```python
from build123d import *

# Parameters (mm, degrees)
F0_W      = 100
F0_H      = 100
F1_DEPTH  = 2
F2_R      = 0.5
F4_W      = 80
F4_H      = 80
F5_DEPTH  = 30
F6_R      = 1
F7_R      = 1
F8_W      = 50
F8_H      = 50
F9_DEPTH  = 20
F10_R     = 1
F11_W     = 40
F11_H     = 40
F12_DEPTH = 42


with BuildPart() as f1:
    # F0 (on Top) → F1 (new body)
    with BuildSketch(Plane.XY):
        Rectangle(F0_W, F0_H)
    extrude(amount=F1_DEPTH)

    # F2
    f2_edges = [f1.edges().sort_by_distance(p)[0] for p in [
        (50, 0, 2),
        (0, 50, 2),
        (-50, 0, 2),
        (0, -50, 2),
    ]]
    fillet(f2_edges, radius=F2_R)

    # F4 (on offset) → F5 (join)
    with BuildSketch(Plane.XY.offset(2)):
        Rectangle(F4_W, F4_H)
    extrude(amount=F5_DEPTH)

    # F6
    f6_edges = [f1.edges().sort_by_distance(p)[0] for p in [
        (-40, -40, 17),
        (40, -40, 17),
        (40, 40, 17),
        (-40, 40, 17),
    ]]
    fillet(f6_edges, radius=F6_R)

    # F7
    f7_edges = [f1.edges().sort_by_distance(p)[0] for p in [
        (40, 0, 32),
        (39.707107, -39.707107, 32),
        (39.707107, 39.707107, 32),
        (0, -40, 32),
        (0, 40, 32),
        (-39.707107, -39.707107, 32),
        (-39.707107, 39.707107, 32),
        (-40, 0, 32),
    ]]
    fillet(f7_edges, radius=F7_R)

    # F8 (on face) → F9 (join)
    with BuildSketch(Plane.XY.offset(32)):
        Rectangle(F8_W, F8_H)
    extrude(amount=F9_DEPTH)

    # F10
    f10_edges = [f1.edges().sort_by_distance(p)[0] for p in [
        (-25, -25, 42),
        (25, -25, 42),
        (0, -25, 32),
        (0, -25, 52),
        (-25, 25, 42),
        (-25, 0, 32),
        (-25, 0, 52),
        (25, 0, 52),
        (0, 25, 52),
        (25, 25, 42),
        (25, 0, 32),
        (0, 25, 32),
    ]]
    fillet(f10_edges, radius=F10_R)

    # F11 (on face) → F12 (cut)
    with BuildSketch(Plane(origin=(0, 0, 0), x_dir=(1, 0, 0), z_dir=(0, 0, -1))):
        Rectangle(F11_W, F11_H)
    extrude(amount=-F12_DEPTH, mode=Mode.SUBTRACT)


solid = f1.part
```
Could you check a few things on this model? Use its own coordinates, in mm. A direction names the side the tool comes from. Coordinates: 2 decimals unless noted, no trailing zeros. Order: outer loops, then holes, each group sorted by start corner. A loop starts at its lowest first (then second) coordinate and runs counter-clockwise, first axis right, second up. Notation, with made-up numbers: M 66,77.5 L 120,77.5 A6 cw 120,82.5 Z; hole C -17,-36 d3. An arc over 180 degrees is marked long. Use a Markdown table: item, result. Add a question column.
Q1. I want a section at A-A on z = 37. List the corners of the cut face in (x, y) for me.
Q2. We'd pull the mould along X, two halves only. Please class faces 6 (the flat face through (0, 20, 21)), 7 (the flat face through (0, 25, 42)), 8 (the flat face through (-25, 0, 42)): pulls with the +X half, pulls with the -X half, needs draft (parallel to the pull), parting line crosses it, or undercut.
Q3. I'm going to push flat-ended pins straight in: pin 1 (14.5 mm diameter, centred on x = 9, z = 41, fed in from -Y); pin 2 (9 mm diameter, centred on y = -8, z = 39, fed in from -X); pin 3 (23 mm diameter, centred on x = -12.5, z = 18.5, fed in from +Y). Where does each tip first touch, or does it pass through?
Q4. If I drill on L1, parallel to X at y = -9, z = 3.5; L2, parallel to X at y = 28.5, z = 12.5, over which ranges is the centre line in solid material (lowest first)?
Q5. I want a section at C-C on y = 16. List the corners of the cut face in (x, z) for me.
Q6. I want a section at B-B on x = -28. List the corners of the cut face in (y, z) for me, then the cut area to 3 significant figures.
Q7. I want a section at D-D on z = 46. List the corners of the cut face in (x, y) for me.
Q8. Which directions (+Z, -Z, +X, -X, +Y, -Y) give clear straight access to the entire face, cutting with the end or side of a thin tool? Please do faces 1 (the flat face through (0, -20, 21)), 2 (the flat face through (0, -25, 42)), 3 (the flat face through (-40, -1, 16)), 4 (the flat face through (25, 0, 42)), 5 (the flat face through (-1, 40, 16)).
Checked values:
| question | item | result |
|---|---|---|
| 1 | outline | M -25,-24 A1 ccw -24,-25 L 24,-25 A1 ccw 25,-24 L 25,24 A1 ccw 24,25 L -24,25 A1 ccw -25,24 Z; hole M -20,-20 L 20,-20 L 20,20 L -20,20 Z |
| 2 | face 6 | undercut |
| 2 | face 7 | needs draft |
| 2 | face 8 | pulls with the -X half |
| 3 | pin 1 | y = -25 |
| 3 | pin 2 | x = -25 |
| 3 | pin 3 | y = 40 |
| 4 | L1 | -40 to -20, 20 to 40 |
| 4 | L2 | -40 to 40 |
| 5 | outline | M -50,0 L -20,0 L -20,42 L 20,42 L 20,0 L 50,0 L 50,1.5 A0.5 ccw 49.5,2 L 40,2 L 40,31 A1 ccw 39,32 L 26,32 A1 cw 25,33 L 25,51 A1 ccw 24,52 L -24,52 A1 ccw -25,51 L -25,33 A1 cw -26,32 L -39,32 A1 ccw -40,31 L -40,2 L -49.5,2 A0.5 ccw -50,1.5 Z |
| 6 | outline | M -50,0 L 50,0 L 50,1.5 A0.5 ccw 49.5,2 L 40,2 L 40,31 A1 ccw 39,32 L -39,32 A1 ccw -40,31 L -40,2 L -49.5,2 A0.5 ccw -50,1.5 Z |
| 6 | area | 2,600 mm² |
| 7 | outline | M -25,-24 A1 ccw -24,-25 L 24,-25 A1 ccw 25,-24 L 25,24 A1 ccw 24,25 L -24,25 A1 ccw -25,24 Z |
| 8 | face 1 | -Z |
| 8 | face 2 | +Z, +X, -X, -Y |
| 8 | face 3 | +Z, -X, +Y, -Y |
| 8 | face 4 | +Z, +X, +Y, -Y |
| 8 | face 5 | +Z, +X, -X, +Y |
